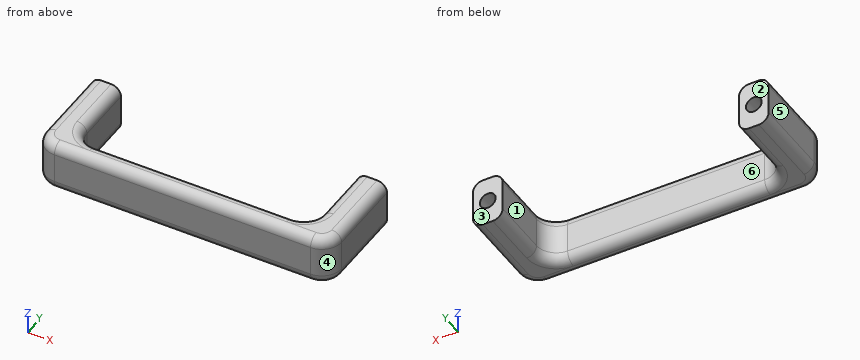
```python
from build123d import *

# Parameters (mm, degrees)
F1_DEPTH = 25
F2_R     = 4.99999
F4_D     = 8
F4_DEPTH = 12
F4_TIP   = 2.4034424761
F6_D     = 8
F6_DEPTH = 12
F6_TIP   = 2.4034424761


# Not quite as in the source:
# - a fillet or chamfer is up to 0.001 mm smaller than in the source, because OpenCascade refuses the exact size


with BuildPart() as f1:
    # F0 (on Top) → F1 (new body)
    with BuildSketch(Plane.XY):
        with BuildLine():
            Line((75, -15), (75, 25))
            Line((75, 25), (60, 25))
            Line((60, 25), (60, -5))
            ThreePointArc((60, -5), (57.0710678119, -12.0710678119), (50, -15))
            Line((50, -15), (-50, -15))
            ThreePointArc((-50, -15), (-57.0710678119, -12.0710678119), (-60, -5))
            Line((-60, -5), (-60, 25))
            Line((-60, 25), (-75, 25))
            Line((-75, 25), (-75, -15))
            ThreePointArc((-75, -15), (-72.0710678119, -22.0710678119), (-65, -25))
            Line((-65, -25), (65, -25))
            ThreePointArc((65, -25), (72.0710678119, -22.0710678119), (75, -15))
        make_face()
    extrude(amount=F1_DEPTH)

    # F2 (radius 5 in the source; OpenCascade refuses exactly that, so slightly less here)
    f2_edges = [f1.edges().sort_by_distance(p)[0] for p in [
        (-57.071068, -12.071068, 0),
        (-57.071068, -12.071068, 25),
        (-72.071068, -22.071068, 0),
        (-72.071068, -22.071068, 25),
    ]]
    fillet(f2_edges, radius=F2_R)

    # F4
    with Locations(Plane(origin=(0, 25, 0), x_dir=(-1, 0, 0), z_dir=(0, 1, 0))):
        with Locations((67.5, 12.5)):
            Hole(F4_D / 2, depth=F4_DEPTH)
            with Locations((0, 0, -(F4_DEPTH + F4_TIP / 2))):  # 118° drill point
                Cone(0, F4_D / 2, F4_TIP, mode=Mode.SUBTRACT)

    # F6
    with Locations(Plane(origin=(0, 25, 0), x_dir=(-1, 0, 0), z_dir=(0, 1, 0))):
        with Locations((-67.5, 12.5)):
            Hole(F6_D / 2, depth=F6_DEPTH)
            with Locations((0, 0, -(F6_DEPTH + F6_TIP / 2))):  # 118° drill point
                Cone(0, F6_D / 2, F6_TIP, mode=Mode.SUBTRACT)


solid = f1.part
```
CAD build for the part. Positions are in the model's coordinates, mm. Face numbers are marked on the shaded views. A direction names the side the tool comes from. Coordinates: 2 decimals unless noted, no trailing zeros. Order: outer loops, then holes, each group sorted by start corner. A loop starts at its lowest first (then second) coordinate and runs counter-clockwise, first axis right, second up. Notation, with made-up numbers: (30.5, 10) -> (83.5, 10) arc R14 ccw to (83.5, 16) -> close; hole circle Ø2 at (59.5, -16). An arc over 180 degrees is marked (long way). Use one line per item in the form item = value. Start each with the question number.
1) Band-saw the part on D-D on z = 7. Give the cut face in (x, y), then the cut area to 3 significant figures.
2) Band-saw the part on A-A on y = 15. Give the cut face in (x, z).
3) Drop flat-ended pins along their axis: pin 1 (5 mm diameter, centred on x = 67.5, z = 12.5, fed in from +Y); pin 2 (12 mm diameter, centred on x = 57.5, y = -5, fed in from +Z); pin 3 (4 mm diameter, centred on x = -28, z = 11.5, fed in from +Y). Give the stop position or say it passes through.
4) Drill centre lines: L1, parallel to X at y = 20.5, z = 12.5; L2, parallel to Z at x = -67.5, y = 18.5; L3, parallel to X at y = 10.5, z = 19.25. Where is each one in solid material? Low to high. Write a range as [from, to].
5) Pull direction X, two halves, no side cores. Call the marked faces 3, 4, 5 and 6: +X half, -X half, draft (parallel to the pull), parting line (faces both ways), or undercut.
6) Band-saw the part on B-B on y = 4. Give the cut face in (x, z).
7) Tool access for the marked faces 1 and 2: list every direction of +Z, -Z, +X, -X, +Y, -Y with a clear straight run to the whole face (end or side of a thin tool).
Entries:
q1.outline = (-75, -15) arc R10 ccw to (-65, -25) -> (65, -25) arc R10 ccw to (75, -15) -> (75, 25) -> (60, 25) -> (60, -5) arc R10 cw to (50, -15) -> (-50, -15) arc R10 cw to (-60, -5) -> (-60, 25) -> (-75, 25) -> close
q1.area = 2,700 mm2
q2.outline = (-75, 5) arc R5 ccw to (-70, 0) -> (-65, 0) arc R5 ccw to (-60, 5) -> (-60, 20) arc R5 ccw to (-65, 25) -> (-70, 25) arc R5 ccw to (-75, 20) -> close; (60, 5) arc R5 ccw to (65, 0) -> (70, 0) arc R5 ccw to (75, 5) -> (75, 20) arc R5 ccw to (70, 25) -> (65, 25) arc R5 ccw to (60, 20) -> close; hole circle Ø8 at (-67.5, 12.5); hole circle Ø8 at (67.5, 12.5)
q3.pin_1 = 12.1
q3.pin_2 = 24.77
q3.pin_3 = -15
q4.L1 = [-75, -71.5], [-63.5, -60], [60, 63.5], [71.5, 75]
q4.L2 = [0, 8.5], [16.5, 25]
q4.L3 = [-75, -60], [60, 75]
q5.face_3 = draft
q5.face_4 = +X half
q5.face_5 = -X half
q5.face_6 = undercut
q6.outline = (-75, 5) arc R5 ccw to (-70, 0) -> (-65, 0) arc R5 ccw to (-60, 5) -> (-60, 20) arc R5 ccw to (-65, 25) -> (-70, 25) arc R5 ccw to (-75, 20) -> close; (60, 5) arc R5 ccw to (65, 0) -> (70, 0) arc R5 ccw to (75, 5) -> (75, 20) arc R5 ccw to (70, 25) -> (65, 25) arc R5 ccw to (60, 20) -> close
q7.face_1 = +Z, -Z, +Y
q7.face_2 = +Z, -Z, +X, -X, +Y
